Could you check a few things on this model? Use its own coordinates, in mm. Face numbers are marked on the shaded views. A direction names the side the tool comes from. Give positions to 0.01 mm unless a question says otherwise; leave off trailing zeros. Loops run counter-clockwise (first coordinate to the right, second up) from the corner with the lowest first, then second, coordinate; pieces in that order, holes last. Notation, with made-up numbers: (-34.75, 21.5) - (-1.75, 21.5) arc R24 cw to (-1.75, 44.5) - close; hole circle Ø4 at (32.25, -31). An arc over 180 degrees is marked (long way). Write each question's results on one line, items separated by ' | '. Start each with the question number.
1) I'm going to push flat-ended pins straight in: pin 1 (10.5 mm diameter, centred on y = 37, z = 40, fed in from +X); pin 2 (11 mm diameter, centred on y = 40, z = 40, fed in from -X); pin 3 (13 mm diameter, centred on y = 41.5, z = 35.5, fed in from -X). Where does each tip first touch, or does it pass through?
2) If I drill on probe 1 along Y at (x, z) = (4.25, 40); probe 2 along Y at (x, z) = (10.7, 40); probe 3 along X at (y, z) = (36, 56.5), over which ranges is the centre line in solid material (lowest first)? Write a range as [from, to].
3) If we mould it in two halves opening along Y, with no side actions, what happens to the marked faces 3, 4 and 5? For each: +Y half, -Y half, draft (parallel to the pull), parting line (faces both ways), or undercut.
4) I want a section at D-D, the plane z = 49.5. Write out the boundary of the cut face in (x, y).
5) On a 3-axis mill with a long thin cutter (end or side, diameter ignored), from which of +Z, -Z, +X, -X, +Y, -Y can I reach the whole of each face in a straight line? I mean the marked faces 1 and 2. Say none if no direction works.
6) I want a section at C-C, the plane x = 5.75. Write out the boundary of the cut face in (y, z).
7) I want a section at A-A, the plane y = 40. Write out the boundary of the cut face in (x, z).
from build123d import *

# Parameters (mm, degrees)
SKETCH_1_W      = 80
SKETCH_1_H      = 80
EXTRUDE_1_DEPTH = 15


with BuildPart() as part:
    # Эскиз1 → Бобышка-Вытянуть1 (new body)
    with BuildSketch(Plane(origin=(0, 0, 0), x_dir=(0, -1, 0), z_dir=(-1, 0, 0))):
        with Locations((-40, 40)):
            Rectangle(SKETCH_1_W, SKETCH_1_H)
    extrude(amount=-EXTRUDE_1_DEPTH)

    # Эскиз2 → Вырез-Повернуть1 (revolve, cut)
    with BuildSketch(Plane(origin=(0, 0, 40), x_dir=(-1, 0, 0), z_dir=(0, 0, -1)), mode=Mode.PRIVATE) as cut_revolve_1_sk:
        Polygon((-15, 57.5), (-15, 40), (0, 40), (0, 53), (-10, 53), (-10, 46), (-13, 46), (-13, 57.5), align=None)
    revolve(cut_revolve_1_sk.sketch.rotate(Axis((15, 40, 40), (-1, 0, 0)), 270), axis=Axis((15, 40, 40), (-1, 0, 0)), mode=Mode.SUBTRACT)


solid = part.part
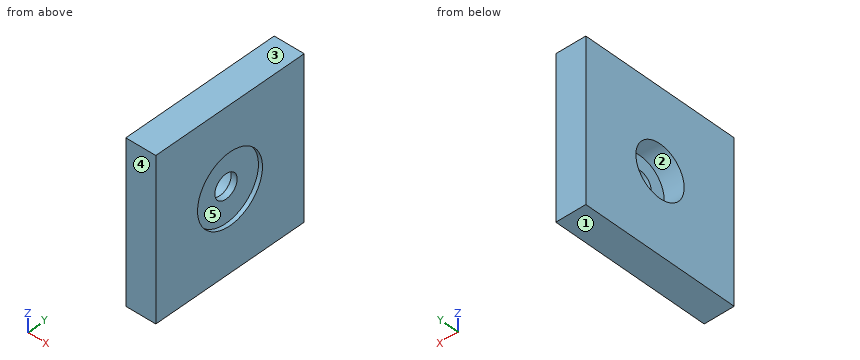
Answers:
1) pin 1: stops at x = 13 | pin 2: passes through | pin 3: stops at x = 10
2) probe 1: y = [0, 27], [53, 80] | probe 2: y = [0, 34], [46, 80] | probe 3: x = [0, 13]
3) face 3: draft | face 4: -Y half | face 5: undercut
4) outline: (0, 0) - (15, 0) - (15, 25.3) - (13, 25.3) - (13, 54.7) - (15, 54.7) - (15, 80) - (0, 80) - (0, 48.87) - (10, 48.87) - (10, 31.13) - (0, 31.13) - close
5) face 1: -Z, +X, -X, +Y, -Y | face 2: -X
6) outline: (0, 0) - (80, 0) - (80, 80) - (0, 80) - close; hole circle Ø26 at (40, 40)
7) outline: (0, 0) - (15, 0) - (15, 22.5) - (13, 22.5) - (13, 34) - (10, 34) - (10, 27) - (0, 27) - close; (0, 53) - (10, 53) - (10, 46) - (13, 46) - (13, 57.5) - (15, 57.5) - (15, 80) - (0, 80) - close
